Geometry: final body of the model. Coordinates: model frame, mm. A direction names the side the tool comes from. Give positions to 0.01 mm unless a question says otherwise; leave off trailing zeros. Loops run counter-clockwise (first coordinate to the right, second up) from the corner with the lowest first, then second, coordinate; pieces in that order, holes last.
1. Section C-C, the plane y = -16. Output: boundary loops of the cut face in (x, z), then the cut area to 3 significant figures.
2. First-contact query: P1, Ø15, axis at x = 7, y = -61, coming from the +Z side; P2, Ø2, axis at x = -11, z = 57, coming from the -Y side. Flat tips, straight axial feed; report the tip coordinate or a pass-through.
3. Section D-D, the plane y = -57. Output: boundary loops of the cut face in (x, z).
4. Material intervals for line 1 along Z through (x, y) = (0, -16); line 2 along X through (y, z) = (-9, 101); line 3 along Z through (x, y) = (-35.5, -62), sorted ascending.
5. Section B-B, the plane x = 0. Output: boundary loops of the cut face in (y, z) (3 decimals), then the cut area to 3 significant figures.
6. Section A-A, the plane z = 101.6. Output: boundary loops of the cut face in (x, y) (3 decimals).
7. Draft query along Z for faces 1 (the face through (-2.48, -23.835, 120.488)), 2 (the face through (1, -39, 0)), 3 (the face through (1, 0, 75)), 4 (the face through (1, -13, 152.4)). Return one class per face: +Z half, -Z half, draft (parallel to the pull), parting line (faces both ways), or undercut.
8. Access query for faces 5 (the face through (76.2, -22, 60)), 6 (the face through (-44, -76.2, 13)), 7 (the face through (1, -50, 25.4)), 8 (the face through (12.4, -22.225, 97.6)), 9 (the face through (12.7, -70, 13)). Directions: +Z, -Z, +X, -X, +Y, -Y. A direction counts if a zero-diameter tool reaches every point of the face in a straight line with its end or side. Return the directions, or none.
from build123d import *

# Parameters (mm, degrees)
F1_DEPTH = 76.2
F2_R     = 12.7
F3_DEPTH = 76.201
F5_DEPTH = 25.401
F6_R     = 19.05
F6_R_2   = 12.7
F7_DEPTH = 3.175


with BuildPart() as f1:
    # F0 (on Right) → F1 (new body, symmetric)
    with BuildSketch(Plane.YZ):
        Polygon((-76.2, 0), (0, 0), (0, 152.4), (-25.4, 152.4), (-25.4, 25.4), (-76.2, 25.4), align=None)
    extrude(amount=F1_DEPTH, both=True)

    # F2 (on face) → F3 (cut, through all)
    with BuildSketch(Plane(origin=(0, 0, 0), x_dir=(-1, 0, 0), z_dir=(0, 1, 0))):
        with Locations((0, 101.6)):
            Circle(F2_R)
    extrude(amount=-F3_DEPTH, mode=Mode.SUBTRACT)

    # F4 (on face) → F5 (cut, through all)
    with BuildSketch(Plane.XY.offset(25.4)):
        with BuildLine():
            Line((-12.7, -63.5), (-12.7, -76.2))
            Line((-12.7, -76.2), (12.7, -76.2))
            Line((12.7, -76.2), (12.7, -63.5))
            ThreePointArc((12.7, -63.5), (0, -50.8), (-12.7, -63.5))
        make_face()
    extrude(amount=-F5_DEPTH, mode=Mode.SUBTRACT)

    # F6 (on face) → F7 (cut, symmetric)
    with BuildSketch(Plane.XZ.offset(25.4)):
        with Locations((0, 101.6)):
            Circle(F6_R)
        with Locations((0, 101.6)):
            Circle(F6_R_2, mode=Mode.SUBTRACT)
    extrude(amount=F7_DEPTH, both=True, mode=Mode.SUBTRACT)


solid = f1.part
Answers below:
1. outline: (-76.2, 0) - (76.2, 0) - (76.2, 152.4) - (-76.2, 152.4) - close; hole circle Ø25.4 at (0, 101.6)
1. area: 22,700 mm2
2. P1: stops at z = 25.4
2. P2: stops at y = -25.4
3. outline: (-76.2, 0) - (-10.91, 0) - (-10.91, 25.4) - (-76.2, 25.4) - close; (10.91, 0) - (76.2, 0) - (76.2, 25.4) - (10.91, 25.4) - close
4. line 1: z = 0 to 88.9, 114.3 to 152.4
4. line 2: x = -76.2 to -12.69, 12.69 to 76.2
4. line 3: z = 0 to 25.4
5. outline: (-50.8, 0) - (0, 0) - (0, 88.9) - (-22.225, 88.9) - (-22.225, 82.55) - (-25.4, 82.55) - (-25.4, 25.4) - (-50.8, 25.4) - close; (-25.4, 120.65) - (-22.225, 120.65) - (-22.225, 114.3) - (0, 114.3) - (0, 152.4) - (-25.4, 152.4) - close
5. area: 3,830 mm2
6. outline: (-76.2, -25.4) - (-19.05, -25.4) - (-19.05, -22.225) - (-12.7, -22.225) - (-12.7, 0) - (-76.2, 0) - close; (12.7, -22.225) - (19.05, -22.225) - (19.05, -25.4) - (76.2, -25.4) - (76.2, 0) - (12.7, 0) - close
7. face 1: undercut
7. face 2: -Z half
7. face 3: draft
7. face 4: +Z half
8. face 5: +Z, -Z, +X, +Y, -Y
8. face 6: +Z, -Z, +X, -X, -Y
8. face 7: +Z, +X, -X, -Y
8. face 8: -Y
8. face 9: +Z, -Z, -Y
